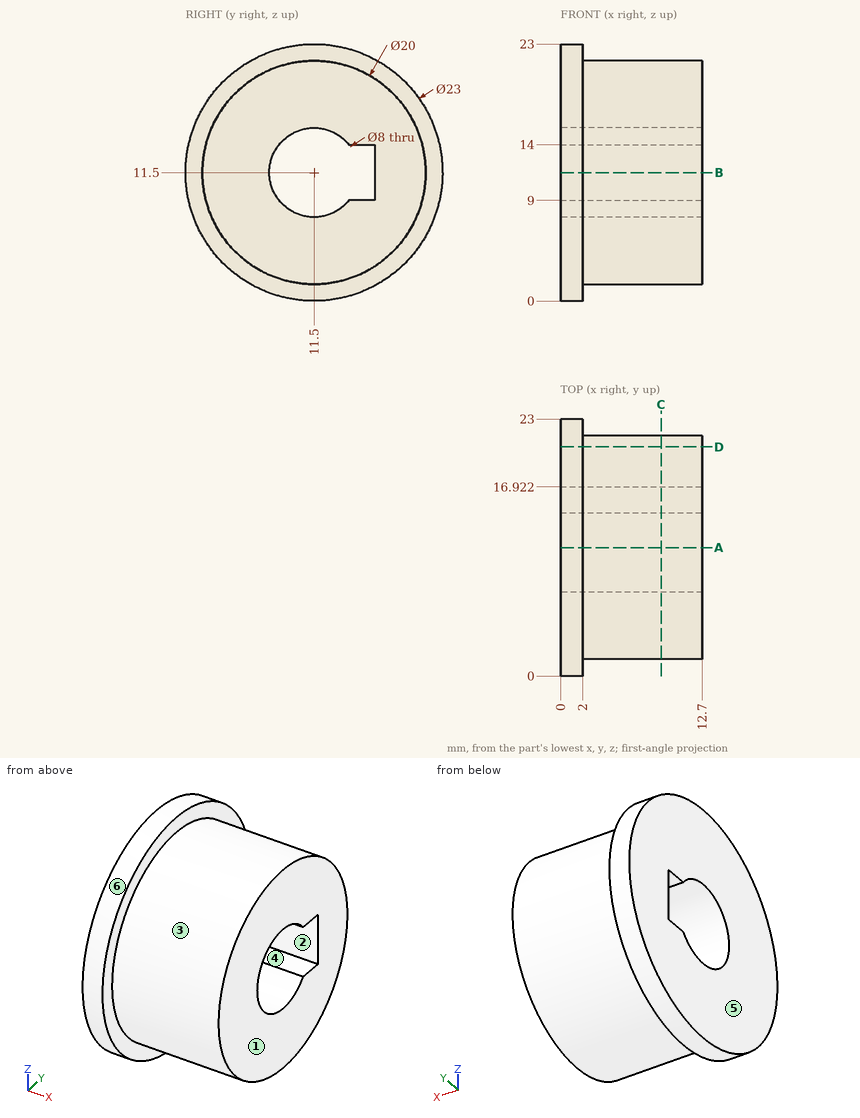
Geometry: see drawing. Coordinates: mm, zero at the bounding-box minimum. A direction names the side the tool comes from. Give positions to 0.01 mm unless a question says otherwise; leave off trailing zeros. Order: outer loops, then holes, each group sorted by start corner. A loop starts at its lowest first (then second) coordinate and runs counter-clockwise, first axis right, second up. Notation, with made-up numbers: (-0.75, 88) - (11.25, 88) arc R19 cw to (11.25, 110) - close; hole circle Ø7 at (68.25, 52). An arc over 180 degrees is marked (long way). Use a Markdown table: item, result.
(1) Section query D-D (y = 20.5). Output: boundary loops of the cut face in (x, z), then the cut area to 3 significant figures.
Computed values:
| item | result |
|---|---|
| outline | (0, 4.34) - (2, 4.34) - (2, 7.14) - (12.7, 7.14) - (12.7, 15.86) - (2, 15.86) - (2, 18.66) - (0, 18.66) - close |
| area | 122 mm2 |
(2) Section query B-B (z = 11.5). Output: boundary loops of the cut face in (x, y).
Computed values:
| item | result |
|---|---|
| outline | (0, 0) - (2, 0) - (2, 1.5) - (12.7, 1.5) - (12.7, 7.5) - (0, 7.5) - close; (0, 16.92) - (12.7, 16.92) - (12.7, 21.5) - (2, 21.5) - (2, 23) - (0, 23) - close |
(3) Draft query along Y for the marked faces 4, 5 and 6. Return one class per face: released by +Y, released by -Y, zero draft, split by the parting line, or undercut.
Computed values:
| item | result |
|---|---|
| face 4 | undercut |
| face 5 | zero draft |
| face 6 | split by the parting line |
(4) Access query for the marked faces 1, 2 and 3. Directions: +Z, -Z, +X, -X, +Y, -Y. A direction counts if a zero-diameter tool reaches every point of the face in a straight line with its end or side. Return the directions, or none.
Computed values:
| item | result |
|---|---|
| face 1 | +Z, -Z, +X, +Y, -Y |
| face 2 | +X, -X |
| face 3 | +X |
(5) Section query A-A (y = 11.5). Output: boundary loops of the cut face in (x, z).
Computed values:
| item | result |
|---|---|
| outline | (0, 0) - (2, 0) - (2, 1.5) - (12.7, 1.5) - (12.7, 7.5) - (0, 7.5) - close; (0, 15.5) - (12.7, 15.5) - (12.7, 21.5) - (2, 21.5) - (2, 23) - (0, 23) - close |
(6) Line query: line 1 (Y direction, x = 6.5, z = 11.5); line 2 (Z direction, x = 9, y = 11.5); line 3 (X direction, y = 1.5, z = 14). Output: solid intervals per line, ascending. Write a range as from..to.
Computed values:
| item | result |
|---|---|
| line 1 | y = 1.5..7.5, 16.92..21.5 |
| line 2 | z = 1.5..7.5, 15.5..21.5 |
| line 3 | x = 0..2 |
(7) Section query C-C (x = 9). Output: boundary loops of the cut face in (y, z), then the cut area to 3 significant figures.
Computed values:
| item | result |
|---|---|
| outline | circle Ø20 at (11.5, 11.5); hole (14.62, 9) - (16.92, 9) - (16.92, 14) - (14.62, 14) arc R4 ccw (long way) to start |
| area | 255 mm2 |
(8) Pin query (flat end, axial travel): pin 1 (2 mm diameter, centred on x = 7, y = 14, fed in from +Z); pin 2 (5 mm diameter, centred on y = 11.5, z = 11.5, fed in from -X); pin 3 (1 mm diameter, centred on x = 5.5, z = 6, fed in from +Y); pin 4 (1 mm diameter, centred on x = 7.5, z = 6, fed in from -Y). Return the tip coordinate at first contact, or that it passes through.
Computed values:
| item | result |
|---|---|
| pin 1 | stops at z = 21.39 |
| pin 2 | passes through |
| pin 3 | stops at y = 20.16 |
| pin 4 | stops at y = 2.84 |
